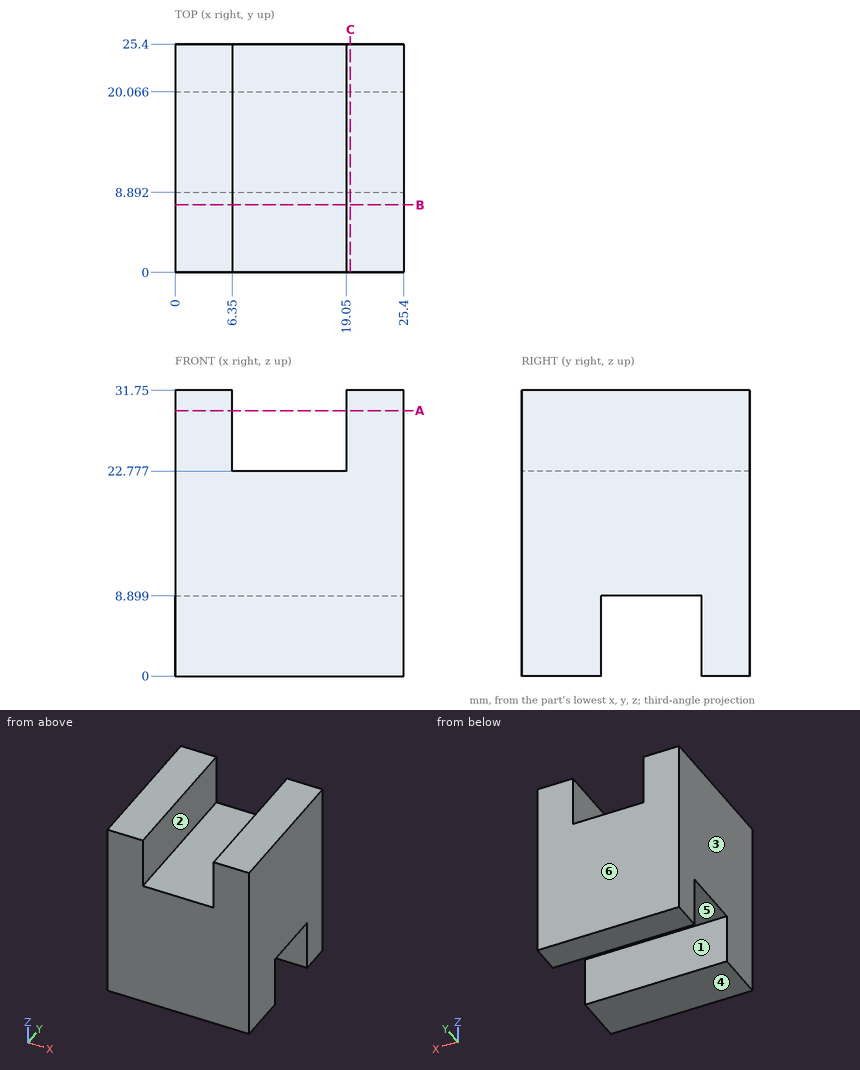
Could you check a few things on this drawing? It's one solid part, dimensions in mm from its lowest x, y, z. A direction names the side the tool comes from. Give positions to 0.01 mm unless a question says otherwise; leave off trailing zeros. Order: outer loops, then holes, each group sorted by start corner. A loop starts at its lowest first (then second) coordinate and runs counter-clockwise, first axis right, second up. Notation, with made-up numbers: M -40,41.5 L 8,41.5 A21 cw 8,73.5 Z; hole C 76,13.5 d8. An arc over 180 degrees is marked long. Use one line per item in the form item = value. Start each with the question number.
Item 1: For the marked faces 1, 2 and 3, which set-ups out of +Z, -Z, +X, -X, +Y, -Y let a thin tool reach every point of the face, with its end or its side?
Item 2: If we section it at C-C (x = 19.5): Write out the boundary of the cut face in (y, z).
Item 3: If we section it at B-B (y = 7.5): Write out the boundary of the cut face in (x, z).
Item 4: If we section it at A-A (z = 29.5): Write out the boundary of the cut face in (x, y).
Item 5: Will these pins go through, and if not, where does the flat tip stop? pin 1 Ø1 at (x, y) = (14, 23) entering from +Z; pin 2 Ø2 at (x, y) = (6, 12.5) entering from -Z.
Item 6: If I drill on line 1 along Y through (x, z) = (15.75, 3.5); line 2 along X through (y, z) = (7, 26.5); line 3 along Z through (x, y) = (19, 23.25), over which ranges is the centre line in solid material (lowest first)?
Item 7: We'd pull the mould along Y, two halves only. Please class the marked faces 4, 5 and 6: +Y half, -Y half, draft (parallel to the pull), parting line (faces both ways), or undercut.
Outcome:
q1.face_1 = -Z, +X, -X
q1.face_2 = +Z, +Y, -Y
q1.face_3 = +Z, -Z, -X, +Y, -Y
q2.outline = M 0,0 L 8.89,0 L 8.89,8.9 L 20.07,8.9 L 20.07,0 L 25.4,0 L 25.4,31.75 L 0,31.75 Z
q3.outline = M 0,0 L 25.4,0 L 25.4,31.75 L 19.05,31.75 L 19.05,22.78 L 6.35,22.78 L 6.35,31.75 L 0,31.75 Z
q4.outline = M 0,0 L 6.35,0 L 6.35,25.4 L 0,25.4 Z; M 19.05,0 L 25.4,0 L 25.4,25.4 L 19.05,25.4 Z
q5.pin_1 = 22.78
q5.pin_2 = 8.9
q6.line_1 = 0 to 8.89, 20.07 to 25.4
q6.line_2 = 0 to 6.35, 19.05 to 25.4
q6.line_3 = 0 to 22.78
q7.face_4 = draft
q7.face_5 = undercut
q7.face_6 = +Y half
